The drawing under review shows one solid part. Ordinate dimensions are in mm from its lowest x, y, z. Give positions to 0.01 mm unless a question says otherwise; leave off trailing zeros. Write each loop counter-clockwise with the first axis right and the second up, starting at its lowest first coordinate (ties: lowest second). Pieces come first, ordered by that corner, then holes. Notation, with made-up numbers: (12.5, -11) -> (44.5, -11) arc R20 ccw to (44.5, -2) -> close; hole circle Ø2 at (9.5, 26). An arc over 180 degrees is marked (long way). Use CSV: the item, a comma, the result in double quotes.
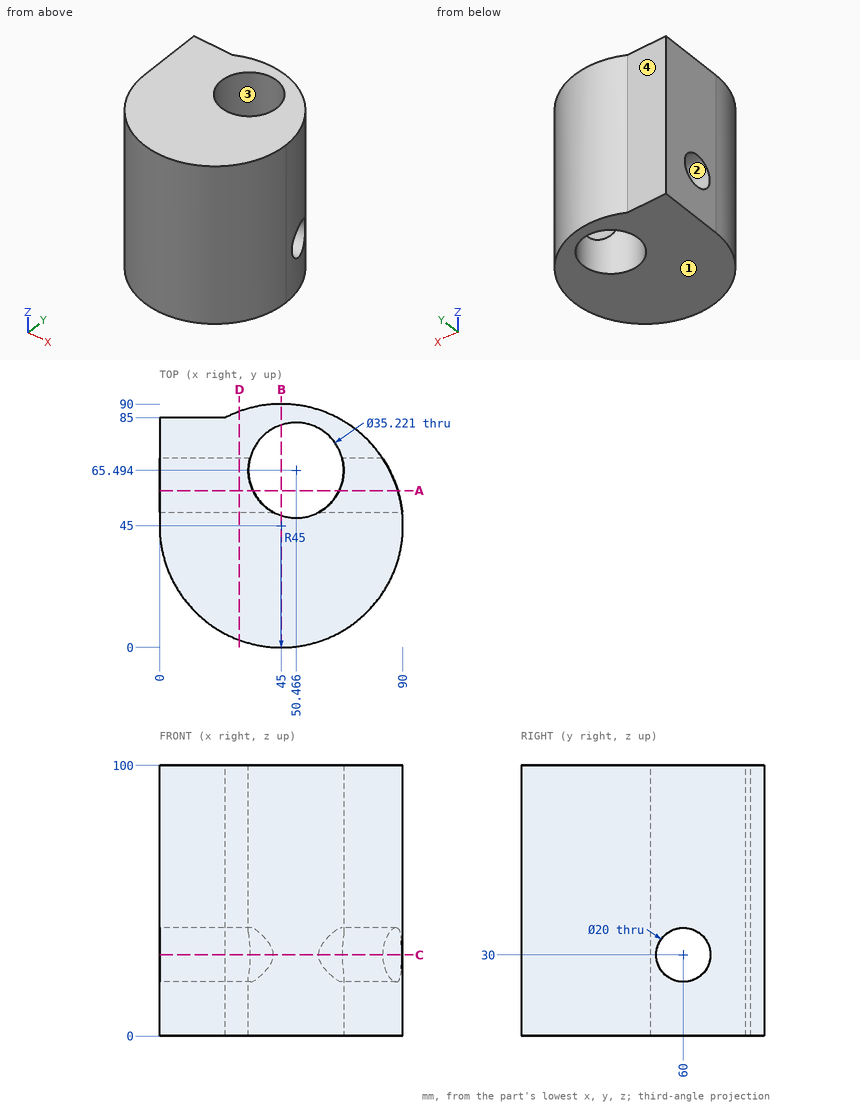
(1) Take a section at B-B (x = 45). Write out the cut boundary in (y, z) (1 decimal), then the cut area to 3 significant figures.
Established:
outline,"(0, 0) -> (48.8, 0) -> (48.8, 100) -> (0, 100) -> close; (82.2, 0) -> (90, 0) -> (90, 100) -> (82.2, 100) -> close"
area,"5,650 mm2"
(2) Take a section at A-A (y = 58). Write out the cut boundary in (x, z), then the cut area to 3 significant figures.
Established:
outline,"(0, 0) -> (34.53, 0) -> (34.53, 20.2) -> (0, 20.2) -> close; (0, 39.8) -> (34.53, 39.8) -> (34.53, 100) -> (0, 100) -> close; (66.4, 0) -> (88.08, 0) -> (88.08, 20.2) -> (66.4, 20.2) -> close; (66.4, 39.8) -> (88.08, 39.8) -> (88.08, 100) -> (66.4, 100) -> close"
area,"4,520 mm2"
(3) Take a section at D-D (x = 29.5). Write out the cut boundary in (y, z), then the cut area to 4 significant figures.
Established:
outline,"(2.75, 0) -> (87.25, 0) -> (87.25, 100) -> (2.75, 100) -> close; hole circle Ø20 at (60, 30)"
area,"8,135 mm2"
(4) For line 1 along Z through (x, y) = (25, 60); line 2 along Y through (x, z) = (39, 92); line 3 along X through (y, z) = (78, 40) (1 decimal), list the stretches that pass through material, from the lowest coordinate up. Write a range as [from, to].
Established:
line 1,"z = [0, 20], [40, 100]"
line 2,"y = [0.4, 52.13], [78.86, 89.6]"
line 3,"x = [0, 38.1], [62.9, 75.6]"
(5) Mouldability with a two-part tool opening along Y and no side actions: class the marked faces 1, 2, 3 and 4 as +Y half, -Y half, draft (parallel to the pull), parting line (faces both ways), or undercut.
Established:
face 1,"draft"
face 2,"undercut"
face 3,"undercut"
face 4,"+Y half"
(6) Clearance check with flat-ended pins moving along their axes: pin 1 (6 mm diameter, centred on x = 65.5, z = 51.5, fed in from +Y); pin 2 (4 mm diameter, centred on y = 23.5, z = 10.5, fed in from -X); pin 3 (5 mm diameter, centred on y = 21.5, z = 22, fed in from -X). State where each tip first meets the part, or that it passes through.
Established:
pin 1,"stops at y = 86.46"
pin 2,"stops at x = 4.44"
pin 3,"stops at x = 5.2"
(7) Take a section at C-C (z = 30). Write out the cut boundary in (x, y), then the cut area to 3 significant figures.
Established:
outline,"(0, 45) arc R45 ccw (long way) to (89.72, 50) -> (58.84, 50) arc R17.61 cw to (42.1, 50) -> (0, 50) -> close; (0, 70) -> (33.44, 70) arc R17.61 cw to (67.49, 70) -> (82.42, 70) arc R45 ccw to (24.38, 85) -> (0, 85) -> close"
area,"4,550 mm2"
